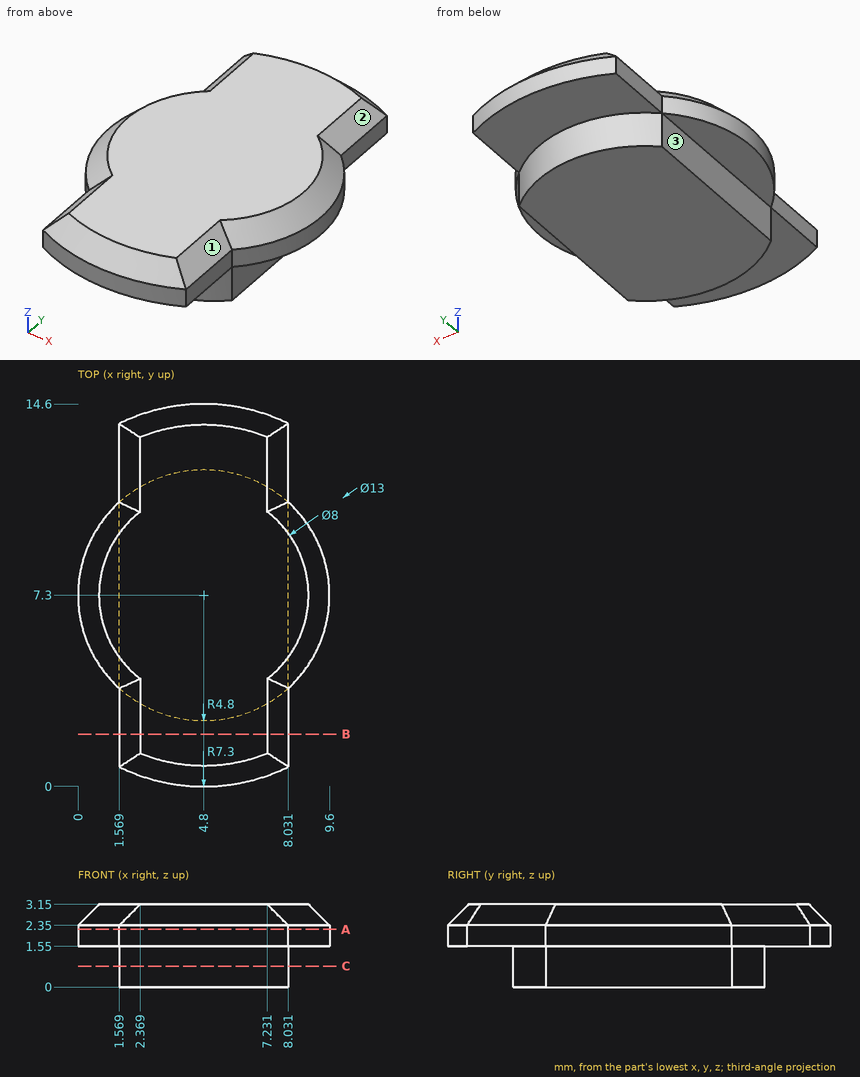
The figure shows three views and two pictorial views of one solid part (mm, origin at its lowest corner). Answer the questions. A direction names the side the tool comes from. Give positions to 0.01 mm unless a question says otherwise; leave off trailing zeros. Write each loop counter-clockwise with the first axis right and the second up, starting at its lowest first coordinate (ties: lowest second). Pieces come first, ordered by that corner, then holes. Notation, with made-up numbers: M -23,-29 L 30,-29 A20 cw 30,6 Z; hole C -23.75,20.25 d2. An arc over 180 degrees is marked long. Write each question's results on one line, items separated by ' | '.
Q1. Section B-B, the plane y = 2 is taken. Write down the section's boundary in (x, z).
Output values:
outline: M 1.57,1.55 L 8.03,1.55 L 8.03,2.35 L 7.23,3.15 L 2.37,3.15 L 1.57,2.35 Z
Q2. Section A-A, the plane z = 2.2 is taken. Write down the section's boundary in (x, y).
Output values:
outline: M 1.57,0.75 A7.3 ccw 8.03,0.75 L 8.03,3.75 A4.8 ccw 8.03,10.85 L 8.03,13.85 A7.3 ccw 1.57,13.85 L 1.57,10.85 A4.8 ccw 1.57,3.75 Z
Q3. Consider L1, parallel to Z at x = 4.25, y = 12.25; L2, parallel to X at y = 3.5, z = 2.2; L3, parallel to Y at x = 8.5, z = 1.65. Determine where each line is inside the solid, lowest interval first. Write a range as from..to.
Output values:
L1: 1.55..3.15 | L2: 1.57..8.03 | L3: 4.24..10.36
Q4. Flat-ended cylindrical pins translate along their axes: P1, Ø0.9, axis at y = 2.5, z = 2, coming from the -X side; P2, Ø0.9, axis at y = 12, z = 2, coming from the +X side; P3, Ø0.8, axis at x = 9, y = 8.5, coming from the -Z side. Find the tip coordinate at first contact, or state that the pin passes through.
Output values:
P1: x = 1.57 | P2: x = 8.03 | P3: z = 1.55
Q5. Section C-C, the plane z = 0.8 is taken. Write down the section's boundary in (x, y).
Output values:
outline: M 1.57,3.75 A4.8 ccw 8.03,3.75 L 8.03,10.85 A4.8 ccw 1.57,10.85 Z
Q6. A tool of negligible diameter and unlimited length cuts with its end or side. For the marked faces 1, 2 and 3, from which of +Z, -Z, +X, -X, +Y, -Y can it reach the whole face along a straight path? Write none if from no direction.
Output values:
face 1: +Z, +X, -Y | face 2: +Z, +X, +Y | face 3: -Z, -X, +Y, -Y
